Could you check a few things on this model? Use its own coordinates, in mm. Round coordinates to 2 decimals unless told otherwise and drop trailing zeros. Loops run counter-clockwise (first coordinate to the right, second up) from the corner with the lowest first, then second, coordinate; pieces in that order, holes last. Notation, with made-up numbers: (38, 10) -> (57, 10) arc R23 cw to (57, 44) -> close; hole circle Ø3 at (37, 28). An arc over 180 degrees is marked (long way). One line per item, written item: value.
```python
from build123d import *

# Parameters (mm, degrees)
SKETCH1_R           = 9.398
BOSS_EXTRUDE1_DEPTH = 6.6802


with BuildPart() as part:
    # Sketch1 → Boss-Extrude1 (new body)
    with BuildSketch(Plane.XY):
        with BuildLine():
            ThreePointArc((67.2719, -2.667), (71.112502584, -1.978843865), (74.475234217, 0))
            Line((74.475234217, 0), (253.108565783, 0))
            ThreePointArc((253.108565783, 0), (256.471297416, -1.978843865), (260.3119, -2.667))
            Line((260.3119, -2.667), (265.43, -2.667))
            ThreePointArc((265.43, -2.667), (296.037, -33.274), (265.43, -63.881))
            Line((265.43, -63.881), (254, -63.881))
            Line((254, -63.881), (254, -78.192462102))
            Line((254, -78.192462102), (258.804744722, -78.192462102))
            ThreePointArc((258.804744722, -78.192462102), (319.641243362, -44.945714973), (330.2, 23.573905719))
            Line((330.2, 23.573905719), (330.2, 44.344229198))
            ThreePointArc((330.2, 44.344229198), (330.227085405, 57.966090028), (316.629665681, 57.15))
            Line((316.629665681, 57.15), (267.494134319, 57.15))
            ThreePointArc((267.494134319, 57.15), (260.3119, 60.515088497), (253.129665681, 57.15))
            Line((253.129665681, 57.15), (113.415260688, 57.15))
            ThreePointArc((113.415260688, 57.15), (86.208048701, 64.123551226), (65.709724775, 83.324632368))
            Line((65.709724775, 83.324632368), (47.058503367, 110.140244689))
            ThreePointArc((47.058503367, 110.140244689), (33.921662387, 117.0051), (20.784821408, 110.140244689))
            Line((20.784821408, 110.140244689), (2.1336, 83.324632368))
            Line((2.1336, 83.324632368), (-4.235992095, 74.166813235))
            ThreePointArc((-4.235992095, 74.166813235), (-5.510617618, 66.127763534), (0, 60.137431006))
            Line((0, 60.137431006), (0, 30.088432035))
            ThreePointArc((0, 30.088432035), (8.908195227, -42.581537647), (73.7489, -76.581))
            ThreePointArc((73.7489, -76.581), (74.974598175, -76.57147033), (76.2, -76.542883623))
            Line((76.2, -76.542883623), (76.2, -63.881))
            Line((76.2, -63.881), (64.77, -63.881))
            ThreePointArc((64.77, -63.881), (34.163, -33.274), (64.77, -2.667))
            Line((64.77, -2.667), (67.2719, -2.667))
        make_face()
        with Locations((33.921662387, 101.0031)):
            Circle(SKETCH1_R, mode=Mode.SUBTRACT)
    extrude(amount=BOSS_EXTRUDE1_DEPTH)


solid = part.part
```
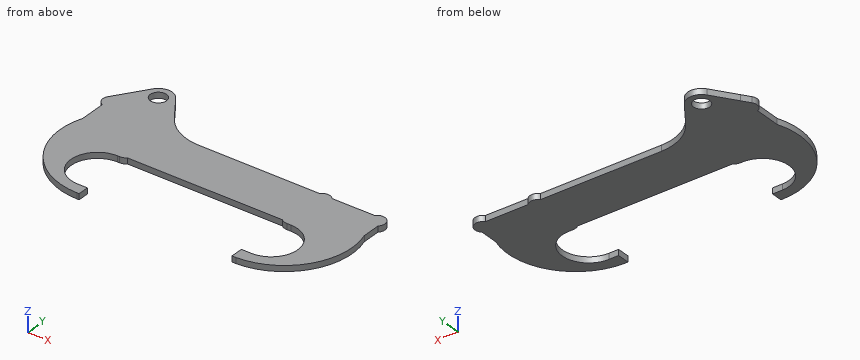
Item 1: If we section it at D-D on x = 147: List the corners of the cut face in (y, z) for me, plus the area to 3 significant figures.
Output:
outline: (0, 0) -> (57.15, 0) -> (57.15, 6.68) -> (0, 6.68) -> close
area: 382 mm²
Item 2: I need wall thicknesses on line 1 (Y direction, x = 173.5, z = 5.25); line 2 (X direction, y = 97, z = 3); line 3 (X direction, y = -67.5, z = 2.75). Which ranges of each line are inside material? Lowest first, please. Write a range as from..to.
Output:
line 1: y = 0..57.15
line 2: x = 11.65..25.42, 42.42..56.2
line 3: x = 37.02..76.2, 254..295.18
Item 3: If we section it at B-B on z = 2.25: List the corners of the cut face in (x, y) for me, plus the area to 3 significant figures.
Output:
outline: (-4.24, 74.17) arc R9.35 ccw to (0, 60.14) -> (0, 30.09) arc R78.83 ccw to (73.75, -76.58) arc R78.83 ccw to (76.2, -76.54) -> (76.2, -63.88) -> (64.77, -63.88) arc R30.61 cw to (64.77, -2.67) -> (67.27, -2.67) arc R11.06 ccw to (74.48, 0) -> (253.11, 0) arc R11.06 ccw to (260.31, -2.67) -> (265.43, -2.67) arc R30.61 cw to (265.43, -63.88) -> (254, -63.88) -> (254, -78.19) -> (258.8, -78.19) arc R78.26 ccw to (330.2, 23.57) -> (330.2, 44.34) arc R9.35 ccw (long way) to (316.63, 57.15) -> (267.49, 57.15) arc R9.35 ccw to (253.13, 57.15) -> (113.42, 57.15) arc R56.56 cw to (65.71, 83.32) -> (47.06, 110.14) arc R16 ccw to (20.78, 110.14) -> close; hole circle Ø18.8 at (33.92, 101)
area: 27,800 mm²
Item 4: Will these pins go through, and if not, where does the flat tip stop? pin 1 Ø1.5 at (x, z) = (276, 5) entering from -Y; pin 2 Ø2 at (x, z) = (291.5, 3.5) entering from +Y; pin 3 Ø3 at (x, z) = (255.5, 4.5) entering from +Y.
Output:
pin 1: stops at y = -75.75
pin 2: stops at y = 57.15
pin 3: stops at y = 59.91
Item 5: If we section it at C-C on y = -52: List the corners of the cut face in (x, z) for me.
Output:
outline: (16.55, 0) -> (40.56, 0) -> (40.56, 6.68) -> (16.55, 6.68) -> close; (289.64, 0) -> (314.06, 0) -> (314.06, 6.68) -> (289.64, 6.68) -> close
Item 6: If we section it at A-A on y = -31: List the corners of the cut face in (x, z) for me.
Output:
outline: (2.27, 0) -> (34.25, 0) -> (34.25, 6.68) -> (2.27, 6.68) -> close; (295.95, 0) -> (327.43, 0) -> (327.43, 6.68) -> (295.95, 6.68) -> close
